Build history of the part. All positions in model axes, mm. Face numbers are marked on the shaded views. A direction names the side the tool comes from. Give positions to 0.01 mm unless a question says otherwise; leave off trailing zeros. Write each loop counter-clockwise with the first axis right and the second up, starting at its lowest first coordinate (ties: lowest second). Pieces come first, ordered by that corner, then holes. Notation, with made-up numbers: (43, 44.5) -> (68, 44.5) arc R29 ccw to (68, 64.5) -> close; hole circle Ø7 at (41, 70.25). An arc over 180 degrees is marked (long way). Put each result on its own line as item: value.
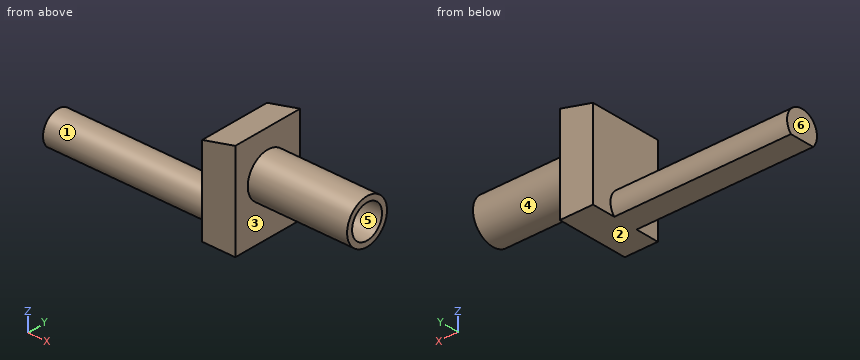
from build123d import *

# Parameters (mm, degrees)
F1_DEPTH  = 20.6375
F2_R      = 9.525
F3_DEPTH  = 50.8
F5_DEPTH  = 127
F7_DEPTH  = 41.276
F8_W      = 41.275
F8_H      = 69.85
F8_R      = 12.7
F9_DEPTH  = 57.15
F10_W     = 25.4
F10_H     = 32.7966427431
F11_DEPTH = 34.926


# Not quite as in the source:
# - a feature names something its author has since deleted; it is built from what else it names


with BuildPart() as f1:
    # F0 (on Front) → F1 (new body, symmetric)
    with BuildSketch(Plane.XZ):
        Polygon((-101.6, -34.925), (101.6, -34.925), (101.6, 34.925), (-101.6, -15.875), align=None)
    extrude(amount=F1_DEPTH, both=True)

    # F2 (on face) → F3 (cut)
    with BuildSketch(Plane.YZ.offset(101.6)):
        with Locations((0, -3.175)):
            Circle(F2_R)
    extrude(amount=-F3_DEPTH, mode=Mode.SUBTRACT)

    # F4 (on face) → F5 (cut)
    with BuildSketch(Plane(origin=(-101.6, 0, 0), x_dir=(0, -1, 0), z_dir=(-1, 0, 0))):
        with BuildLine():
            ThreePointArc((-7.0995158286, -34.925), (0, -19.05), (7.0995158286, -34.925))
            Line((7.0995158286, -34.925), (20.6375, -34.925))
            Line((20.6375, -34.925), (20.6375, -15.875))
            Line((20.6375, -15.875), (-20.6375, -15.875))
            Line((-20.6375, -15.875), (-20.6375, -34.925))
            Line((-20.6375, -34.925), (-7.0995158286, -34.925))
        make_face()
    extrude(amount=-F5_DEPTH, mode=Mode.SUBTRACT)

    # F6 (on face) → F7 (cut, through all)
    with BuildSketch(Plane(origin=(0, 20.6375, 0), x_dir=(-1, 0, 0), z_dir=(0, 1, 0))):
        Polygon((-25.4, 15.875), (-25.4, -15.875), (101.6, -15.875), align=None)
    extrude(amount=-F7_DEPTH, mode=Mode.SUBTRACT)

    # F8 (on face) → F9 (cut)
    with BuildSketch(Plane.YZ.offset(101.6)):
        Rectangle(F8_W, F8_H)
        with Locations((0, -3.175)):
            Circle(F8_R, mode=Mode.SUBTRACT)
    extrude(amount=-F9_DEPTH, mode=Mode.SUBTRACT)

    # F10 (on Top) → F11 (cut, through all)
    with BuildSketch(Plane.XY):
        with Locations((-88.9, -1.6974383034)):
            Rectangle(F10_W, F10_H)
    extrude(amount=-F11_DEPTH, mode=Mode.SUBTRACT)


solid = f1.part
1) Slice it at A-A (z = -1.5). Write the cut outline in (x, y), plus the area to 3 significant figures.
Filled sheet:
outline: (25.4, -20.64) -> (44.45, -20.64) -> (44.45, -12.59) -> (101.6, -12.59) -> (101.6, -9.38) -> (50.8, -9.38) -> (50.8, 9.38) -> (101.6, 9.38) -> (101.6, 12.59) -> (44.45, 12.59) -> (44.45, 20.64) -> (25.4, 20.64) -> close
area: 1,270 mm2
2) Wall check: L1, parallel to Z at x = 91.5, y = 0 (3 decimals); L2, parallel to X at y = 2, z = 10.5; L3, parallel to X at y = 1.5, z = -2.5. Give the ranges that are in metal, low to high.
Filled sheet:
L1: -15.875 to -12.7, 6.35 to 9.525
L2: 25.4 to 44.45
L3: 25.4 to 50.8
3) Slice it at C-C (x = 83.5). Write the cut outline in (y, z) (3 decimals).
Filled sheet:
outline: circle Ø25.4 at (0, -3.175); hole circle Ø19.05 at (0, -3.175)
4) Pin check, flat tips, straight feed: pin 1 (2 mm diameter, centred on y = 5, z = 2.5, fed in from +X); pin 2 (12 mm diameter, centred on x = 75, z = 14, fed in from -Y); pin 3 (2 mm diameter, centred on y = -6.5, z = -14.5, fed in from -X). Stop position of each tip, or through.
Filled sheet:
pin 1: x = 50.8
pin 2: y = -6.03
pin 3: x = 25.4
5) Pull direction Z, two halves, no side cores. Call the marked faces 4, 5 and 6: released by +Z, released by -Z, zero draft, split by the parting line, or undercut.
Filled sheet:
face 4: split by the parting line
face 5: undercut
face 6: zero draft
6) Tool access for the marked faces 1, 2 and 3: list every direction of +Z, -Z, +X, -X, +Y, -Y with a clear straight run to the whole face (end or side of a thin tool).
Filled sheet:
face 1: -X
face 2: -Z, +X, -X, +Y, -Y
face 3: +X
